```python
from build123d import *

# Parameters (mm, degrees)
F0_W     = 98.2365459204
F0_H     = 38.1
F1_DEPTH = 5.08
F3_DEPTH = 25.4


# Not quite as in the source:
# - a feature names something its author has since deleted; it is built from what else it names


with BuildPart() as f1:
    # F0 (on Top) → F1 (new body)
    with BuildSketch(Plane.XY):
        with Locations((0.2698786557, -21.017140013)):
            Rectangle(F0_W, F0_H)
    extrude(amount=F1_DEPTH)

    # F2 (on face) → F3 (cut)
    with BuildSketch(Plane.XY.offset(5.08)):
        with BuildLine():
            Line((-37.191967051, -1.967140013), (-46.9076386285, -1.967140013))
            ThreePointArc((-46.9076386285, -1.967140013), (-42.0498028398, -5.2410121524), (-37.191967051, -1.967140013))
        make_face()
        with BuildLine():
            ThreePointArc((-37.191967051, -1.967140013), (-36.9054766067, -1.0020558812), (-36.8087906874, 0))
            ThreePointArc((-36.8087906874, 0), (-43.051858721, 5.1443262331), (-46.9076386285, -1.967140013))
            Line((-46.9076386285, -1.967140013), (-37.191967051, -1.967140013))
        make_face()
    extrude(amount=-F3_DEPTH, mode=Mode.SUBTRACT)


solid = f1.part
```
The model under review builds one solid part; all positions refer to its coordinate system, in mm. Round coordinates to 2 decimals unless told otherwise and drop trailing zeros. Loops run counter-clockwise (first coordinate to the right, second up) from the corner with the lowest first, then second, coordinate; pieces in that order, holes last. Notation, with made-up numbers: M 53,38.25 L 91,38.25 A25 ccw 91,54.25 Z; hole C 84,55 d5. An arc over 180 degrees is marked long. Put each result on its own line as item: value.
Q1. Consider section A-A, the plane x = -43. Give the boundary of the cut face in (y, z).
Result set:
outline: M -40.07,0 L -5.15,0 L -5.15,5.08 L -40.07,5.08 Z
Q2. Mouldability with a two-part tool opening along X and no side actions: class faces 1 (the flat face through (49.388, -21, 3)), 2 (the cylindrical face through (-42.14, -5.24, 2.58)), 3 (the flat face through (-48.848, -21, 3)), 4 (the flat face through (0, -21, 0)) as released by +X, released by -X, zero draft, split by the parting line, or undercut.
Result set:
face 1: released by +X
face 2: undercut
face 3: released by -X
face 4: zero draft
Q3. To check wall thickness, follow L1, parallel to Y at x = -45, z = 2.5; L2, parallel to Y at x = -41, z = 4.75. State the ranges of each line that lie inside material, in increasing order.
Result set:
L1: y = -40.07 to -4.33
L2: y = -40.07 to -5.13
